```python
from build123d import *

# Parameters (mm, degrees)
BOSS_EXTRUDE1_DEPTH = 114.3


with BuildPart() as part:
    # Sketch1 → Boss-Extrude1 (new body, symmetric)
    with BuildSketch(Plane(origin=(0, 0, 0), x_dir=(0, 0, -1), z_dir=(1, 0, 0))):
        with BuildLine():
            Line((-25.3365, -76.2), (-25.3365, 76.2))
            Line((-25.3365, 76.2), (29.5275, 76.2))
            Line((29.5275, 76.2), (29.5275, 73.710744653))
            ThreePointArc((29.5275, 73.710744653), (28.795909131, 71.72969626), (26.952334163, 70.699643218))
            Line((26.952334163, 70.699643218), (-9.856185406, 64.919590337))
            ThreePointArc((-9.856185406, 64.919590337), (-14.465122828, 62.344457732), (-16.2941, 57.391836749))
            Line((-16.2941, 57.391836749), (-16.2941, -57.391836749))
            ThreePointArc((-16.2941, -57.391836749), (-14.465122828, -62.344457732), (-9.856185406, -64.919590337))
            Line((-9.856185406, -64.919590337), (26.952334163, -70.699643218))
            ThreePointArc((26.952334163, -70.699643218), (28.795909131, -71.72969626), (29.5275, -73.710744653))
            Line((29.5275, -73.710744653), (29.5275, -76.2))
            Line((29.5275, -76.2), (-25.3365, -76.2))
        make_face()
    extrude(amount=BOSS_EXTRUDE1_DEPTH, both=True)


solid = part.part
```
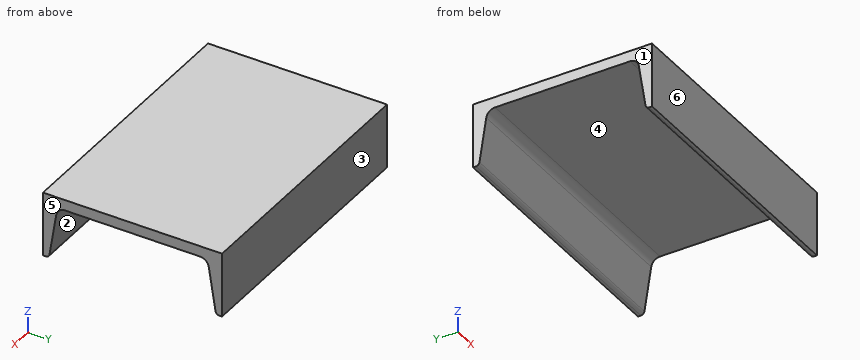
Read the model definition and answer for the solid it produces. Units are mm, in the model's axes. Face numbers are marked on the shaded views. A direction names the side the tool comes from. Round coordinates to 2 decimals unless told otherwise and drop trailing zeros. Write each loop counter-clockwise with the first axis right and the second up, starting at its lowest first coordinate (ties: lowest second). Pieces come first, ordered by that corner, then holes. Notation, with made-up numbers: (42.5, 40.25) - (72.5, 40.25) arc R16 ccw to (72.5, 49.25) - close; hole circle Ø5 at (76.5, 47). An arc over 180 degrees is marked (long way). One line per item, written item: value.
Q1. For a pull along Y with two mould halves and no side action, classify the marked faces 3, 4, 5 and 6 as pulls with the +Y half, pulls with the -Y half, needs draft (parallel to the pull), parting line crosses it, or undercut.
The answers:
face 3: pulls with the +Y half
face 4: undercut
face 5: needs draft
face 6: pulls with the -Y half
Q2. Straight lines are drawn through the part: line 1 (Z direction, x = -37, y = -28); line 2 (Y direction, x = 86, z = 2.5); line 3 (Y direction, x = -38, z = -23). For each, find the intervals that lie inside material, in ascending order. Write a range as from..to.
The answers:
line 1: z = 16.29..25.34
line 2: y = -76.2..-66.07, 66.07..76.2
line 3: y = -76.2..-70.08, 70.08..76.2
Q3. Find section A-A (x = -22). Determine the outline of the cut face in (y, z).
The answers:
outline: (-76.2, -29.53) - (-73.71, -29.53) arc R3.05 ccw to (-70.7, -26.95) - (-64.92, 9.86) arc R7.62 cw to (-57.39, 16.29) - (57.39, 16.29) arc R7.62 cw to (64.92, 9.86) - (70.7, -26.95) arc R3.05 ccw to (73.71, -29.53) - (76.2, -29.53) - (76.2, 25.34) - (-76.2, 25.34) - close
Q4. Which of the six approach directions +Z, -Z, +X, -X, +Y, -Y give full straight-line access (tool end or side, diameter ignored) to the marked faces 1 and 2?
The answers:
face 1: +Z, -Z, -X, +Y, -Y
face 2: -Z, +X, -X
Q5. Find section C-C (y = -19). Determine the outline of the cut face in (x, z).
The answers:
outline: (-114.3, 16.29) - (114.3, 16.29) - (114.3, 25.34) - (-114.3, 25.34) - close
Q6. Find section B-B (z = -14). Determine the outline of the cut face in (x, y), and give its area (3 significant figures).
The answers:
outline: (-114.3, -76.2) - (114.3, -76.2) - (114.3, -68.67) - (-114.3, -68.67) - close; (-114.3, 68.67) - (114.3, 68.67) - (114.3, 76.2) - (-114.3, 76.2) - close
area: 3,440 mm2
